Could you check a few things on this model? Use its own coordinates, in mm. Face numbers are marked on the shaded views. Give positions to 0.01 mm unless a question says otherwise; leave off trailing zeros. Write each loop counter-clockwise with the first axis right and the second up, starting at its lowest first coordinate (ties: lowest second). Pieces come first, ordered by that corner, then holes. Notation, with made-up numbers: M 26,66.25 L 30,66.25 A9 ccw 30,73.25 Z; hole C -18.75,-39.5 d9. An arc over 180 degrees is marked long. Use one line per item in the form item = value.
Autodesk Inventor part; units mm, degrees
ref_plane "YZ Plane" through (0, 0, 0) normal (1, 0, 0) x (0, 1, 0)
ref_plane "XZ Plane" through (0, 0, 0) normal (0, 1, 0) x (-1, 0, 0)
ref_plane "XY Plane" through (0, 0, 0) normal (0, 0, 1) x (1, 0, 0)
sketch "Boceto1" plane through (0, 0, 0) normal (0, 1, 0) x (-1, 0, 0)
  circle A0 centre (0, 0) radius 62.862
  circle A1 centre (0, 0) radius 52.5
  dimension "d0" = 125.724
  dimension "d1" = 105
extrude "Extrusión1" add sketch "Boceto1" along normal blind 23
sketch "Boceto2" plane through (0, 23, 0) normal (0, 1, 0) x (1, 0, 0)
  circle A0 centre (0, 0) radius 52.5
extrude "Extrusión2" add sketch "Boceto2" against normal blind 5
sketch "Boceto3" plane through (0, 23, 0) normal (0, 1, 0) x (1, 0, 0)
  circle A0 centre (0, 0) radius 2.65
  dimension "d6" = 5.3
extrude "Extrusión3" cut sketch "Boceto3" against normal through all
sketch "Boceto4" plane through (0, 23, 0) normal (0, 1, 0) x (1, 0, 0)
  circle A0 centre (-59.612, 0) radius 1.65
  point P0 (0, 0)
  dimension "d9" = 3.3
  dimension "d10" = 59.612
extrude "Extrusión4" cut sketch "Boceto4" against normal through all
pattern_circular "Patrón circular1" count 12 over 360 about axis through (0, 0, 0) along (0, 1, 0) of "Extrusión4"
fillet "Empalme1" radius 3 1 edges at (52.5, 18, 0)
sketch "Boceto6" plane through (0, 23, 0) normal (0, 1, 0) x (1, 0, 0)
  circle A0 centre (0, -59.612) radius 1.65
  circle A1 centre (0, -59.612) radius 2.85
  line L0 (1.6454, -62.462) -> (-1.6454, -62.462)
  line L1 (-1.6454, -62.462) -> (-3.2909, -59.612)
  line L2 (-3.2909, -59.612) -> (-1.6454, -56.762)
  line L3 (-1.6454, -56.762) -> (1.6454, -56.762)
  line L4 (1.6454, -56.762) -> (3.2909, -59.612)
  line L5 (3.2909, -59.612) -> (1.6454, -62.462)
  point P0 (0, 0)
  dimension "d20" = 5.7
extrude "Extrusión6" [suppressed]
pattern_circular "Patrón circular2" [suppressed]
sketch "Boceto10" plane through (0, 0, 0) normal (0, -1, 0) x (1, 0, 0)
  circle A0 centre (0, 0) radius 2.65
  circle A1 centre (0, 0) radius 81.3362
extrude "Extrusión10" cut sketch "Boceto10" against normal blind 16.5
sketch "Boceto11" plane through (0, 23, 0) normal (0, 1, 0) x (1, 0, 0)
  circle A0 centre (0, -20) radius 2.7
  circle A1 centre (0, -40) radius 2.7
  point P0 (0, 0)
  dimension "d40" = 5.4
  dimension "d41" = 20
  dimension "d42" = 20
extrude "Extrusión11" cut sketch "Boceto11" against normal through all
sketch "Boceto12" plane through (0, 18, 0) normal (0, -1, 0) x (1, 0, 0)
  circle A0 centre (0, 0) radius 2.65
  circle A1 centre (0, 0) radius 5
  circle A2 centre (0, 20) radius 2.7
  circle A3 centre (0, 20) radius 5
  circle A4 centre (0, 40) radius 2.7
  circle A5 centre (0, 40) radius 5
  dimension "d45" = 10
extrude "Extrusión12" cut sketch "Boceto12" against normal blind 2 contours A0 | A1 | A2 | A3 | A4 | A5
sketch "Boceto9" plane through (0, 18, 0) normal (0, -1, 0) x (1, 0, 0)
  circle A0 centre (0, 0) radius 2.65
  circle A1 centre (0, 0) radius 74.2803
sketch "Boceto8" plane through (0, 0, 0) normal (0, -1, 0) x (1, 0, 0)
  circle A0 centre (0, 0) radius 2.65
  circle A1 centre (0, 0) radius 69.5586
sketch "Boceto7" plane through (0, 0, 0) normal (0, -1, 0) x (1, 0, 0)
  line L0 (0, 0) -> (-67.2382, 47.1765)
  line L1 (-67.2382, 47.1765) -> (-46.5407, 66.6024)
  circle A0 centre (0, 0) radius 2.65
  line L2 (-46.5407, 66.6024) -> (0, 0)
  line L3 (0, 0) -> (-86.5562, 0)
  line L4 (0, 0) -> (-56.8894, 56.8894)
  point P0 (-1.5179, 2.1722)
  point P1 (-2.1693, 1.5221)
  dimension "d26" = 20
  dimension "d28" = 45
properties part number "Platform"
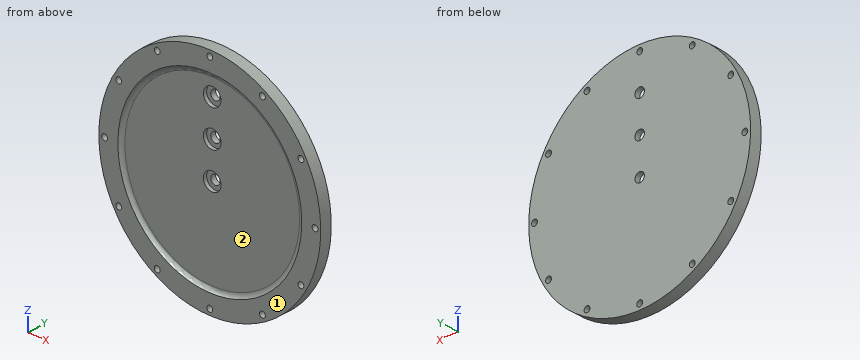
1) Thinking about a two-plate mould opening in Z: for the marked faces 1 and 2, which applies, released by +Z, released by -Z, zero draft, split by the parting line, or undercut?
Checked values:
face_1 = zero draft
face_2 = undercut
2) I want a section at B-B, the plane x = 0. Count the separate pieces of the cut face and the enclosed holes in it, plus the area to 3 significant figures.
Checked values:
separate_pieces = 6
enclosed_holes = 0
area = 512 mm2
3) If I drill on L1, parallel to X at y = 19.5, z = 52.5; L2, parallel to Y at x = 38.5, z = -10.5; L3, parallel to Z at x = -31, y = 19.5, over which ranges is the centre line in solid material (lowest first)?
Checked values:
L1 = -34.57 to -31.21, -28.41 to 28.41, 31.21 to 34.57
L2 = 18 to 23
L3 = -54.69 to -52.76, -50.49 to 50.49, 52.76 to 54.69
4) I want a section at A-A, the plane z = 0. Please give me the cut outline in (x, y), plus the area to 3 significant figures.
Checked values:
outline = M -62.86,16.5 L -61.26,16.5 L -61.26,23 L -62.86,23 Z; M -57.96,16.5 L -52.1,16.5 A3 cw -49.5,18 L -5,18 L -5,20 L -2.65,20 L -2.65,23 L -57.96,23 Z; M 2.65,20 L 5,20 L 5,18 L 49.5,18 A3 cw 52.1,16.5 L 57.96,16.5 L 57.96,23 L 2.65,23 Z; M 61.26,16.5 L 62.86,16.5 L 62.86,23 L 61.26,23 Z
area = 584 mm2
5) For pin 1 Ø4 at (x, z) = (-51.63, -29.81) entering from +Y; pin 2 Ø1 at (x, z) = (36.5, -2) entering from -Y; pin 3 Ø2.5 at (x, z) = (29.81, 51.63) entering from -Y; pin 4 Ø3 at (y, z) = (20.5, -48) entering from -X, each with a flat end and sliding along its axis, tell me the tip position at first contact or that it passes through.
Checked values:
pin_1 = 23
pin_2 = 18
pin_3 = through
pin_4 = -42.3
